```python
from build123d import *

# Parameters (mm, degrees)
SKETCH1_R               = 233.4
SKETCH1_R_2             = 152.4
BOSS_EXTRUDE1_DEPTH     = 45
SKETCH2_R               = 152.4
BOSS_EXTRUDE2_DEPTH     = 12.5
FILLET2_R               = 10
FILLET3_R               = 10
FILLET4_R               = 10
SKETCH3_R               = 13
SKETCH3_R_2             = 6
CUT_EXTRUDE2_DEPTH      = 46
CUT_EXTRUDE2_DEPTH_BACK = 46


with BuildPart() as part:
    # Sketch1 → Boss-Extrude1 (new body, symmetric)
    with BuildSketch(Plane(origin=(0, 0, 0), x_dir=(0, 0, -1), z_dir=(1, 0, 0))):
        Circle(SKETCH1_R)
        Circle(SKETCH1_R_2, mode=Mode.SUBTRACT)
    extrude(amount=BOSS_EXTRUDE1_DEPTH, both=True)

    # Sketch2 → Boss-Extrude2 (add, symmetric)
    with BuildSketch(Plane(origin=(0, 0, 0), x_dir=(0, 0, -1), z_dir=(1, 0, 0))):
        Circle(SKETCH2_R)
    extrude(amount=BOSS_EXTRUDE2_DEPTH, both=True)

    # Fillet2
    fillet2_edges = [part.edges().sort_by_distance(p)[0] for p in [
        (45, 0, 233.4),
    ]]
    fillet(fillet2_edges, radius=FILLET2_R)

    # Fillet3
    fillet3_edges = [part.edges().sort_by_distance(p)[0] for p in [
        (-45, 0, 233.4),
        (45, 0, 152.4),
    ]]
    fillet(fillet3_edges, radius=FILLET3_R)

    # Fillet4
    fillet4_edges = [part.edges().sort_by_distance(p)[0] for p in [
        (-45, 0, 152.4),
    ]]
    fillet(fillet4_edges, radius=FILLET4_R)

    # Sketch3 → Cut-Extrude2 (cut, two sides)
    with BuildSketch(Plane(origin=(0, 0, 0), x_dir=(0, 0, -1), z_dir=(1, 0, 0))) as cut_extrude2_sk:
        Circle(SKETCH3_R)
        with Locations((30, 40)):
            Circle(SKETCH3_R_2)
        with Locations((-30, 40)):
            Circle(SKETCH3_R_2)
        with Locations((-30, -40)):
            Circle(SKETCH3_R_2)
        with Locations((30, -40)):
            Circle(SKETCH3_R_2)
    extrude(amount=CUT_EXTRUDE2_DEPTH, mode=Mode.SUBTRACT)
    extrude(cut_extrude2_sk.sketch, amount=-CUT_EXTRUDE2_DEPTH_BACK, mode=Mode.SUBTRACT)


solid = part.part
```
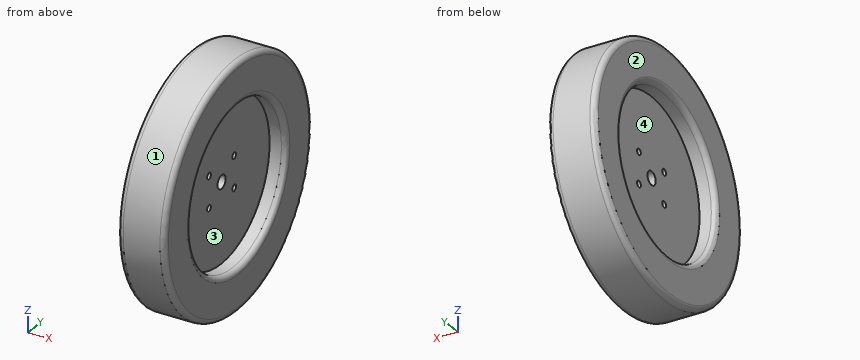
CAD build for the part. Positions are in the model's coordinates, mm. Face numbers are marked on the shaded views. Coordinates: 2 decimals unless noted, no trailing zeros. Order: outer loops, then holes, each group sorted by start corner. A loop starts at its lowest first (then second) coordinate and runs counter-clockwise, first axis right, second up. Notation, with made-up numbers: (-19.5, 28) - (0.5, 28) arc R30 ccw to (0.5, 52) - close; hole circle Ø2 at (76.25, 66). An arc over 180 degrees is marked (long way). Use a Markdown table: item, result. Add a question column.
(1) Flat gauge pins, fed straight in: pin 1 (5 mm diameter, centred on x = -7.5, y = 44, fed in from +Z); pin 2 (5 mm diameter, centred on x = 7, y = 153.5, fed in from +Z); pin 3 (10 mm diameter, centred on x = 22.5, z = 57.5, fed in from +Y). Where does each tip first touch, or does it go through?
(2) Saw through at A-A (y = 0). Give the cut face in (x, z).
(3) Saw through at C-C (z = -30). Count the separate pieces of the cut face and the enclosed holes in it, then the cut area to 3 significant figures.
(4) Drill centre lines: line 1 along Y through (x, z) = (3, 0); line 2 along Y through (x, z) = (-29.5, 0); line 3 along X through (y, z) = (-54, 119.5). Where is each one in solid material? Low to high. Write a range as [from, to].
(5) Saw through at B-B (x = -1). Give the cut face in (y, z).
(6) Pull direction Z, two halves, no side cores. Call the marked faces 1, 2, 3 and 4: +Z half, -Z half, draft (parallel to the pull), parting line (faces both ways), or undercut.
Solved:
| question | item | result |
|---|---|---|
| 1 | pin 1 | stops at z = 229.68 |
| 1 | pin 2 | stops at z = 177.97 |
| 1 | pin 3 | stops at y = 227.42 |
| 2 | outline | (-45, -223.4) arc R10 ccw to (-35, -233.4) - (35, -233.4) arc R10 ccw to (45, -223.4) - (45, -162.4) arc R10 ccw to (35, -152.4) - (12.5, -152.4) - (12.5, -13) - (-12.5, -13) - (-12.5, -152.4) - (-35, -152.4) arc R10 ccw to (-45, -162.4) - close; (-45, 162.4) arc R10 ccw to (-35, 152.4) - (-12.5, 152.4) - (-12.5, 13) - (12.5, 13) - (12.5, 152.4) - (35, 152.4) arc R10 ccw to (45, 162.4) - (45, 223.4) arc R10 ccw to (35, 233.4) - (-35, 233.4) arc R10 ccw to (-45, 223.4) - close |
| 3 | separate pieces | 3 |
| 3 | enclosed holes | 0 |
| 3 | area | 21,500 mm² |
| 4 | line 1 | y = [-233.4, -13], [13, 233.4] |
| 4 | line 2 | y = [-233.4, -152.4], [152.4, 233.4] |
| 4 | line 3 | x = [-12.5, 12.5] |
| 5 | outline | circle Ø466.8 at (0, 0); hole circle Ø12 at (-40, -30); hole circle Ø12 at (-40, 30); hole circle Ø26 at (0, 0); hole circle Ø12 at (40, -30); hole circle Ø12 at (40, 30) |
| 6 | face 1 | parting line |
| 6 | face 2 | draft |
| 6 | face 3 | undercut |
| 6 | face 4 | undercut |
